Autodesk Inventor part; units mm, degrees
ref_plane "YZ Plane" through (0, 0, 0) normal (1, 0, 0) x (0, 1, 0)
ref_plane "XZ Plane" through (0, 0, 0) normal (0, 1, 0) x (-1, 0, 0)
ref_plane "XY Plane" through (0, 0, 0) normal (0, 0, 1) x (1, 0, 0)
sketch "Sketch1" plane through (0, 0, 0) normal (0, 1, 0) x (-1, 0, 0)
  line L0 (0, 0) -> (57.15, 0)
  line L1 (112.534, 31.2241) -> (58.0687, -3.175)
  line L2 (58.0687, -3.175) -> (0, -3.175)
  line L3 (0, -3.175) -> (0, 0)
  line L4 (110.8385, 33.9086) -> (112.534, 31.2241)
  line L5 (57.15, 0) -> (110.8385, 33.9086)
  dimension "d0" = 3.175
  dimension "d1" = 3.175
  dimension "d3" = 57.15
  dimension "d4" = 63.5
  dimension "d5" = 147.724
extrude "Extrusion1" add sketch "Sketch1" along normal blind 25.4
sketch "Sketch2" plane through (-57.15, 0, 0) normal (0, 0, 1) x (1, 0, 0)
  line L0 (0, 25.4) -> (57.15, 25.4)
  circle A0 centre (57.15, 25.4) radius 11.1125
  line L1 (57.15, 0) -> (57.15, 25.4)
  circle A1 centre (57.15, 25.4) radius 19.05
  dimension "d8" = 22.225
  dimension "d9" = 38.1
extrude "Extrusion2" add sketch "Sketch2" against normal blind 3.175 contours A1 L1 A0 L0 | L0 A0 L1 A1
sketch "Sketch3" plane through (-57.15, 0, 0) normal (0, 0, 1) x (1, 0, 0)
  line L0 (57.15, 14.2875) -> (57.15, 25.4)
  circle A0 centre (57.15, 25.4) radius 11.1125
  point P0 (57.15, 0)
extrude "Extrusion3" cut sketch "Sketch3" against normal blind 3.175
fillet "Fillet1" radius 3.175 2 edges at (0, 6.35, -1.5875) (-19.05, 25.4, -1.5875)
sketch "Sketch4" plane through (0, 25.4, 0) normal (0, 1, 0) x (1, 0, 0)
  line L0 (0, 0) -> (-63.5, 0)
  line L1 (-136.491, 61.8746) -> (-57.15, 61.8746)
  line L2 (-57.15, 61.8746) -> (-57.15, -40.3817)
  line L3 (-57.15, -40.3817) -> (-136.491, -40.3817)
  line L4 (-136.491, -40.3817) -> (-136.491, 61.8746)
  dimension "d15" = 63.5
extrude "Extrusion4" cut sketch "Sketch4" against normal blind 31.75
sketch "Sketch5" plane through (0, 25.4, 0) normal (0, 1, 0) x (1, 0, 0)
  line L0 (0, 0) -> (-57.15, 0)
  line L1 (-57.15, 0) -> (-57.15, 3.175)
  line L2 (-57.15, 0) -> (-53.975, 0)
  line L3 (-53.975, 0) -> (-53.975, 57.15)
  line L4 (-53.975, 57.15) -> (-57.15, 57.15)
  line L5 (-57.15, 57.15) -> (-57.15, 0)
  dimension "d18" = 57.15
  dimension "d19" = 3.175
  dimension "d20" = 57.15
extrude "Extrusion5" add sketch "Sketch5" against normal up to surface (25.4 mm away)
properties part number "Pivot Bracket"
Design review of the part built by this model. Coordinates are the model's own, in mm. A direction names the side the tool comes from. Coordinates: 2 decimals unless noted, no trailing zeros. Order: outer loops, then holes, each group sorted by start corner. A loop starts at its lowest first (then second) coordinate and runs counter-clockwise, first axis right, second up. Notation, with made-up numbers: (85.5, 49.25) -> (104.5, 49.25) arc R22 cw to (104.5, 81.25) -> close; hole circle Ø6 at (16, 14). An arc over 180 degrees is marked (long way). Use one line per item in the form item = value. Start each with the question number.
(1) Add section A-A on x = -4.5. State the section outline as (y, z) points (3 decimals), plus the area to 3 significant figures.
(2) For probe 1 along X at (y, z) = (25, -2); probe 2 along Z at (x, y) = (-13.5, 22.5) (3 decimals); probe 3 along X at (y, z) = (5, -36.5) (3 decimals), list the stretches that pass through material, from the lowest coordinate up.
(3) Add section B-B on y = 20. State the section outline as (x, z) points (3 decimals), plus the area to 3 significant figures.
(4) Add section D-D on x = 4.5. State the section outline as (y, z) points (3 decimals), plus the area to 3 significant figures.
(5) Insertion check: pin 1 (7.5 mm diameter, centred on y = 6.5, z = -28, fed in from +X) (3 decimals); pin 2 (4 mm diameter, centred on x = -5, y = 15.5, fed in from -Z) (3 decimals); pin 3 (4 mm diameter, centred on x = -10, y = 34.5, fed in from +Z); pin 4 (2.5 mm diameter, centred on y = 1, z = -2, fed in from +X). Each pin has a flat end and moves straight along its axis. Give the tip position at first contact, or say it passes through.
(6) Add section C-C on z = -18. State the section outline as (x, y) points (3 decimals), plus the area to 3 significant figures.
(7) The part is to be moulded in two halves that separate along X. For faces 1 (the flat face through (-57.15, 13, -29)), 2 (the flat face through (-18, 17, -3.175)), 3 (the flat face through (0, 2, -2)), 4 (the cylindrical face through (1.447, 14.382, -1.565)), say which applies: +X half, -X half, draft (parallel to the pull), parting line (faces both ways), or undercut.
(8) For faces 5 (the flat face through (-55, 25.4, -16)), 6 (the cylindrical face through (13.88, 38.45, -1.57)), 7 (the flat face through (-53.975, 13, -30)), list the 3-axis set-ups (+Z, -Z, +X, -X, +Y, -Y) from which the entire face can be reached by the end or side of a thin tool; tool diameter is ignored.
Answer block:
q1.outline = (0, -3.175) -> (15.239, -3.175) -> (15.239, 0) -> (0, 0) -> close; (35.561, -3.175) -> (43.911, -3.175) -> (43.911, 0) -> (35.561, 0) -> close
q1.area = 74.9 mm²
q2.probe_1 = -57.15 to -11.11, 11.11 to 19.05
q2.probe_2 = -3.175 to 0
q2.probe_3 = -57.15 to -53.975
q3.outline = (-57.15, -57.15) -> (-53.975, -57.15) -> (-53.975, -3.175) -> (-9.712, -3.175) -> (-9.712, 0) -> (-57.15, 0) -> close; (9.712, -3.175) -> (18.269, -3.175) -> (18.269, 0) -> (9.712, 0) -> close
q3.area = 349 mm²
q4.outline = (6.889, -3.175) -> (15.239, -3.175) -> (15.239, 0) -> (6.889, 0) -> close; (35.561, -3.175) -> (43.911, -3.175) -> (43.911, 0) -> (35.561, 0) -> close
q4.area = 53.0 mm²
q5.pin_1 = -53.975
q5.pin_2 = -3.175
q5.pin_3 = 0
q5.pin_4 = 0
q6.outline = (-57.15, 0) -> (-53.975, 0) -> (-53.975, 25.4) -> (-57.15, 25.4) -> close
q6.area = 80.6 mm²
q7.face_1 = -X half
q7.face_2 = draft
q7.face_3 = +X half
q7.face_4 = undercut
q8.face_5 = +Z, -Z, -X, +Y
q8.face_6 = +Z, -Z
q8.face_7 = -Z, +X, +Y, -Y
